Verification items for the finished model (mm, model axes). A direction names the side the tool comes from. Give positions to 0.01 mm unless a question says otherwise; leave off trailing zeros. Write each loop counter-clockwise with the first axis right and the second up, starting at its lowest first coordinate (ties: lowest second). Pieces come first, ordered by that corner, then holes. Notation, with made-up numbers: (-14.5, -7) -> (-1.5, -7) arc R9 cw to (-1.5, -2) -> close; hole circle Ø9 at (-7.75, -10.75). An arc over 180 degrees is marked (long way). Answer as CSV lines item,"result". Start each with the question number.
1) Tool access check on faces 1 (the flat face through (37, 0, 40.375)), 2 (the flat face through (-37, 0, 45.015)), 3 (the cylindrical face through (21.082, 0.992, 61.722)), 4 (the flat face through (-33.02, 0, 20)), 5 (the flat face through (37, 0, 45.015)). Record the directions out of +Z, -Z, +X, -X, +Y, -Y that give a thin tool (end or side, any length) a straight path to the whole face; none if there is none.
2) Sectioned sample at C-C on z = 51.5. Record the cut outline in (x, y), and give its area (3 significant figures).
3) Mould release check, pull along X, two halves, no side actions. Record for faces 6 (the flat face through (41.275, 0, 43)), 7 (the flat face through (18, 0, 58.477)), 8 (the cylindrical face through (19.363, 0.451, 61.608)), 9 (the flat face through (1, -15.24, 29)): released by +X, released by -X, zero draft, split by the parting line, or undercut.
4) Gauge pin test, flat ends, axial feed: pin 1 Ø11 at (y, z) = (2, 51) entering from +X; pin 2 Ø6.5 at (x, y) = (-38.77, 7.62) entering from +Z; pin 3 Ø8 at (y, z) = (-12, 17) entering from -X. Record the tip position at first contact, or that the pin passes through.
5) Sectioned sample at B-B on x = -26.5. Record the cut outline in (y, z), and give its area (3 significant figures).
6) Material ranges on L1, parallel to X at y = 11, z = 36.5; L2, parallel to Z at x = 22, y = 3.5; L3, parallel to Z at x = 10, y = -9, recorded low to high.
```python
from build123d import *

# Parameters (mm, degrees)
SKETCH_1_W       = 66.04
SKETCH_1_H       = 30.48
EXTRUDE_1_DEPTH  = 40.3754
EXTRUDE_11_DEPTH = 4.64
SKETCH_3_W       = 66.06472
SKETCH_3_H       = 30.48
EXTRUDE_12_DEPTH = 13.462
SKETCH_5_R       = 6.731
SKETCH_5_R_2     = 3.302
EXTRUDE_13_DEPTH = 0.22537
SKETCH_6_R       = 3.302
SKETCH_6_R_2     = 1.5
EXTRUDE_14_DEPTH = 6.35


with BuildPart() as part:
    # 스케치1 → 보스-돌출1 (new body)
    with BuildSketch(Plane.XY):
        Rectangle(SKETCH_1_W, SKETCH_1_H)
    extrude(amount=EXTRUDE_1_DEPTH)

    # 스케치2 → 보스-돌출11 (add)
    with BuildSketch(Plane.XY.offset(40.3754)):
        with BuildLine():
            Line((41.275, -8.74168445), (41.275, -15.24))
            Line((41.275, -15.24), (-41.275, -15.24))
            Line((-41.275, -15.24), (-41.275, -8.74168445))
            ThreePointArc((-41.275, -8.74168445), (-36.01612, -7.61562), (-41.275, -6.48955555))
            Line((-41.275, -6.48955555), (-41.275, 6.48955555))
            ThreePointArc((-41.275, 6.48955555), (-36.01612, 7.61562), (-41.275, 8.74168445))
            Line((-41.275, 8.74168445), (-41.275, 15.24))
            Line((-41.275, 15.24), (41.275, 15.24))
            Line((41.275, 15.24), (41.275, 8.74168445))
            ThreePointArc((41.275, 8.74168445), (36.01612, 7.61562), (41.275, 6.48955555))
            Line((41.275, 6.48955555), (41.275, -6.48955555))
            ThreePointArc((41.275, -6.48955555), (36.01612, -7.61562), (41.275, -8.74168445))
        make_face()
    extrude(amount=EXTRUDE_11_DEPTH)

    # 스케치3 → 보스-돌출12 (add)
    with BuildSketch(Plane.XY.offset(45.0154)):
        Rectangle(SKETCH_3_W, SKETCH_3_H)
    extrude(amount=EXTRUDE_12_DEPTH)

    # 스케치5 → 보스-돌출13 (add)
    with BuildSketch(Plane.XY.offset(58.4774)):
        with Locations((17.9325, 0)):
            Circle(SKETCH_5_R)
        with Locations((17.9325, 0)):
            Circle(SKETCH_5_R_2, mode=Mode.SUBTRACT)
    extrude(amount=EXTRUDE_13_DEPTH)

    # 스케치6 → 보스-돌출14 (add)
    with BuildSketch(Plane.XY.offset(58.4774)):
        with Locations((17.9325, 0)):
            Circle(SKETCH_6_R)
        with Locations((17.9325, 0)):
            Circle(SKETCH_6_R_2, mode=Mode.SUBTRACT)
    extrude(amount=EXTRUDE_14_DEPTH)


solid = part.part
```
Ans:
1,face 1,"-Z, +X, +Y, -Y"
1,face 2,"+Z, -X, +Y, -Y"
1,face 3,"+Z"
1,face 4,"-Z, -X, +Y, -Y"
1,face 5,"+Z, +X, +Y, -Y"
2,outline,"(-33.03, -15.24) -> (33.03, -15.24) -> (33.03, 15.24) -> (-33.03, 15.24) -> close"
2,area,"2,010 mm²"
3,face 6,"released by +X"
3,face 7,"undercut"
3,face 8,"undercut"
3,face 9,"zero draft"
4,pin 1,"stops at x = 33.03"
4,pin 2,"stops at z = 45.02"
4,pin 3,"stops at x = -33.02"
5,outline,"(-15.24, 0) -> (15.24, 0) -> (15.24, 58.48) -> (-15.24, 58.48) -> close"
5,area,"1,780 mm²"
6,L1,"x = -33.02 to 33.02"
6,L2,"z = 0 to 58.7"
6,L3,"z = 0 to 58.48"
